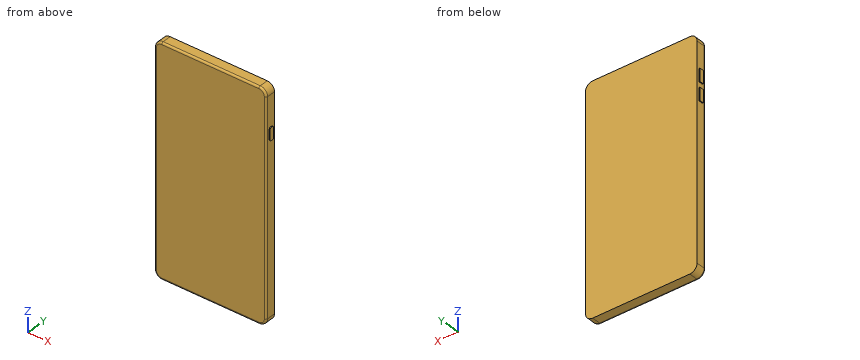
from build123d import *

# Parameters (mm, degrees)
F1_DEPTH = 7.366
F2_R     = 1.27
F4_DEPTH = 0.635
F5_W     = 3.048
F5_H     = 8.89
F6_DEPTH = 0.635


with BuildPart() as f1:
    # F0 (on Front) → F1 (new body)
    with BuildSketch(Plane.XZ):
        with BuildLine():
            Line((0, 153.162), (0, 5.08))
            ThreePointArc((0, 5.08), (1.487898, 1.487898), (5.08, 0))
            Line((5.08, 0), (72.898, 0))
            ThreePointArc((72.898, 0), (76.490102, 1.487898), (77.978, 5.08))
            Line((77.978, 5.08), (77.978, 153.162))
            ThreePointArc((77.978, 153.162), (76.490102, 156.754102), (72.898, 158.242))
            Line((72.898, 158.242), (5.08, 158.242))
            ThreePointArc((5.08, 158.242), (1.487898, 156.754102), (0, 153.162))
        make_face()
    extrude(amount=F1_DEPTH)

    # F2
    f2_edges = [f1.edges().sort_by_distance(p)[0] for p in [
        (38.989, -7.366, 0),
    ]]
    fillet(f2_edges, radius=F2_R)

    # F3 (on face) → F4 (join)
    with BuildSketch(Plane.YZ.offset(77.978)):
        with BuildLine():
            Line((-2.658174, 131.647782), (-3.674174, 131.647782))
            ThreePointArc((-3.674174, 131.647782), (-4.392594, 131.350203), (-4.690174, 130.631782))
            Line((-4.690174, 130.631782), (-4.690174, 123.773782))
            ThreePointArc((-4.690174, 123.773782), (-4.392594, 123.055362), (-3.674174, 122.757782))
            Line((-3.674174, 122.757782), (-2.658174, 122.757782))
            ThreePointArc((-2.658174, 122.757782), (-1.939753, 123.055362), (-1.642174, 123.773782))
            Line((-1.642174, 123.773782), (-1.642174, 130.631782))
            ThreePointArc((-1.642174, 130.631782), (-1.939753, 131.350203), (-2.658174, 131.647782))
        make_face()
    extrude(amount=F4_DEPTH)

    # F5 (on face) → F6 (join)
    with BuildSketch(Plane(origin=(0, 0, 0), x_dir=(0, -1, 0), z_dir=(-1, 0, 0))):
        with Locations((3.230303, 131.321728)):
            Rectangle(F5_W, F5_H)
        with Locations((3.230303, 118.621728)):
            Rectangle(F5_W, F5_H)
    extrude(amount=F6_DEPTH)


solid = f1.part
Could you check a few things on this model? Use its own coordinates, in mm. Round coordinates to 2 decimals unless told otherwise and drop trailing zeros. Write each loop counter-clockwise with the first axis right and the second up, starting at its lowest first coordinate (ties: lowest second). Pieces come first, ordered by that corner, then holes. Notation, with made-up numbers: (50, 5) - (67, 5) arc R14 cw to (67, 12) - close; hole circle Ø6 at (-10.75, -20). An arc over 180 degrees is marked (long way). Use a Markdown table: item, result.
Q1. I want a section at A-A (z = 58). List the corners of the cut face in (x, y) for me.
Output values:
| item | result |
|---|---|
| outline | (0, -6.1) arc R1.27 ccw to (1.27, -7.37) - (76.71, -7.37) arc R1.27 ccw to (77.98, -6.1) - (77.98, 0) - (0, 0) - close |
Q2. Please list where these lines run through material, in increasing order: L1, parallel to X at y = -5.5, z = 51.5; L2, parallel to X at y = -3.75, z = 134 (3 decimals); L3, parallel to Z at x = 73, y = -4.25.
Output values:
| item | result |
|---|---|
| L1 | 0 to 77.98 |
| L2 | -0.635 to 77.978 |
| L3 | 0 to 158.24 |
Q3. For pin 1 (0.7 mm diameter, centred on x = -0.5, y = -2.5, fed in from +Z); pin 2 (1.8 mm diameter, centred on y = -3, z = 58.5, fed in from +X); pin 3 (1.5 mm diameter, centred on y = -2.5, z = 69.5, fed in from -X), each with a flat end and sliding along its axis, tell me the tip position at first contact or that it passes through.
Output values:
| item | result |
|---|---|
| pin 1 | z = 135.77 |
| pin 2 | x = 77.98 |
| pin 3 | x = 0 |
